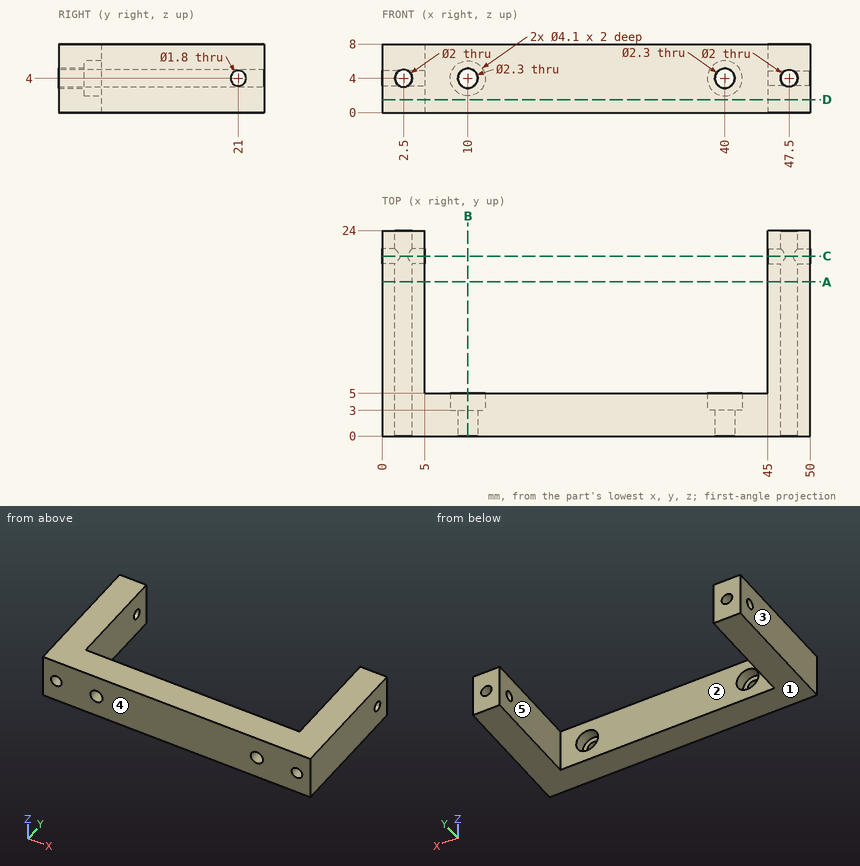
Design review of the part shown in the three views and the two pictorial views. Dimensions are in mm from the part's minimum x, y and z. A direction names the side the tool comes from. Round coordinates to 2 decimals unless told otherwise and drop trailing zeros. Loops run counter-clockwise (first coordinate to the right, second up) from the corner with the lowest first, then second, coordinate; pieces in that order, holes last. Notation, with made-up numbers: M 11,58 L 16,58 A34 cw 16,94 Z; hole C -35,34 d4. An arc over 180 degrees is marked long. Answer as a JSON object with one key per item and string values.
Item 1: Clearance check with flat-ended pins moving along their axes: P1, Ø2.5, axis at x = 10, z = 4, coming from the +Y side; P2, Ø3.5, axis at x = 40.5, z = 3, coming from the +Y side. State where each tip first meets the part, or that it passes through.
Check sheet entries:
{"P1": "y = 3", "P2": "y = 5"}
Item 2: We need section D-D, the plane z = 1.5. State the section outline as (x, y) points.
Check sheet entries:
{"outline": "M 0,0 L 50,0 L 50,24 L 45,24 L 45,5 L 5,5 L 5,24 L 0,24 Z"}
Item 3: For line 1 along X through (y, z) = (4.55, 4); line 2 along X through (y, z) = (13.75, 0.5); line 3 along Y through (x, z) = (4.6, 4), list the stretches that pass through material, from the lowest coordinate up.
Check sheet entries:
{"line 1": "0 to 1.5, 3.5 to 7.95, 12.05 to 37.95, 42.05 to 46.5, 48.5 to 50", "line 2": "0 to 5, 45 to 50", "line 3": "0 to 20.1, 21.9 to 24"}
Item 4: We need section C-C, the plane y = 21. State the section outline as (x, z) points, and give its area (3 significant figures).
Check sheet entries:
{"outline": "M 0,0 L 5,0 L 5,3.1 L 2.94,3.1 A1 cw 2.06,3.1 L 0,3.1 Z; M 0,4.9 L 2.06,4.9 A1 cw 2.94,4.9 L 5,4.9 L 5,8 L 0,8 Z; M 45,0 L 50,0 L 50,3.1 L 47.94,3.1 A1 cw 47.06,3.1 L 45,3.1 Z; M 45,4.9 L 47.06,4.9 A1 cw 47.94,4.9 L 50,4.9 L 50,8 L 45,8 Z", "area": "61.8 mm2"}
Item 5: We need section A-A, the plane y = 18. State the section outline as (x, z) points, and give its area (3 significant figures).
Check sheet entries:
{"outline": "M 0,0 L 5,0 L 5,8 L 0,8 Z; M 45,0 L 50,0 L 50,8 L 45,8 Z; hole C 2.5,4 d2; hole C 47.5,4 d2", "area": "73.7 mm2"}
Item 6: We need section B-B, the plane x = 10. State the section outline as (y, z) points.
Check sheet entries:
{"outline": "M 0,0 L 5,0 L 5,1.95 L 3,1.95 L 3,2.85 L 0,2.85 Z; M 0,5.15 L 3,5.15 L 3,6.05 L 5,6.05 L 5,8 L 0,8 Z"}
Item 7: Tool access review of the marked faces 1 and 2: name each direction out of +Z, -Z, +X, -X, +Y, -Y from which nothing blocks a thin tool from reaching the whole face with its end or side.
Check sheet entries:
{"face 1": "-Z, +X, -X, +Y, -Y", "face 2": "+Z, -Z, +Y"}
Item 8: The part is to be moulded in two halves that separate along X. For the marked faces 3, 4 and 5, say which applies: +X half, -X half, draft (parallel to the pull), parting line (faces both ways), or undercut.
Check sheet entries:
{"face 3": "-X half", "face 4": "draft", "face 5": "undercut"}
